from build123d import *

# Parameters (mm, degrees)
CUT_EXTRUDE1_DEPTH      = 36.362195916
CUT_EXTRUDE1_DEPTH_BACK = 36.362195916
CUT_EXTRUDE2_DEPTH      = 36.362195916
CUT_EXTRUDE2_DEPTH_BACK = 36.362195916
SKETCH4_R               = 4.245


with BuildPart() as part:
    # Sketch1 → Revolve1 (revolve)
    with BuildSketch(Plane(origin=(0, 0, 0), x_dir=(1, 0, 0), z_dir=(0, 1, 0)), mode=Mode.PRIVATE) as revolve1_sk:
        Polygon((-14, -7.07), (-14, 7.07), (-18, 7.07), (-18, 5.5), (-24.5, 5.5), (-24.5, 3.93), (-18, 3.93), (-18, 2.36), (-24.5, 2.36), (-24.5, -2.36), (-18, -2.36), (-18, -3.93), (-24.5, -3.93), (-24.5, -5.5), (-18, -5.5), (-18, -7.07), align=None)
    revolve(revolve1_sk.sketch.rotate(Axis((0, 0, 0), (0, 0, -1)), 180), axis=Axis((0, 0, 0), (0, 0, -1)))

    # Sketch3 → Cut-Extrude1 (cut, two sides: drawn at the far end of the back side and taken through both)
    with BuildSketch(Plane.XY.offset(-CUT_EXTRUDE1_DEPTH_BACK)):
        with BuildLine():
            Line((-14, 0), (-24.5, 0))
            ThreePointArc((-24.5, 0), (0, -24.5), (24.5, 0))
            Line((24.5, 0), (14, 0))
            ThreePointArc((14, 0), (0, -14), (-14, 0))
        make_face()
    extrude(amount=CUT_EXTRUDE1_DEPTH + CUT_EXTRUDE1_DEPTH_BACK, mode=Mode.SUBTRACT)

    # Sketch4 → Cut-Extrude2 (cut, two sides: drawn at the far end of the back side and taken through both)
    with BuildSketch(Plane(origin=(0, 0, 0), x_dir=(1, 0, 0), z_dir=(0, 1, 0)).offset(-CUT_EXTRUDE2_DEPTH_BACK)):
        with Locations(Location((0, 0, 0), (0, 0, 90))):
            Circle(SKETCH4_R)
    extrude(amount=CUT_EXTRUDE2_DEPTH + CUT_EXTRUDE2_DEPTH_BACK, mode=Mode.SUBTRACT)

    # Sketch6 → Tap Drill for M2x0.4 Tap1 (revolve, cut)
    with BuildSketch(Plane(origin=(-21.25, 0, 0), x_dir=(0, 0, -1), z_dir=(1, 0, 0))):
        Polygon((0, 0), (0, 7.2), (1.1, 6.564914704), (1.1, 0), align=None)
    tap_drill_for_m2x0_4_tap1 = revolve(axis=Axis((-21.25, -6.35, 0), (0, 1, 0)), mode=Mode.SUBTRACT)

    # Mirror1: Tap Drill for M2x0.4 Tap1 across plane
    add(tap_drill_for_m2x0_4_tap1.mirror(Plane(origin=(0, 0, 0), x_dir=(0, 0, 1), z_dir=(1, 0, 0))), mode=Mode.SUBTRACT)


solid = part.part
Can you work these out from the model? Positions are in its coordinate system, mm. A direction names the side the tool comes from. Coordinates: 2 decimals unless noted, no trailing zeros. Write each loop counter-clockwise with the first axis right and the second up, starting at its lowest first coordinate (ties: lowest second). Pieces come first, ordered by that corner, then holes. Notation, with made-up numbers: (76, 10.25) -> (80, 10.25) arc R28 cw to (80, 49.25) -> close; hole circle Ø9 at (-2.75, 77.5). An arc over 180 degrees is marked (long way). Write item = value, one per line.
(1) Imagine slicing it at B-B (y = 23). Please give me the cut outline in (x, z) (3 decimals), and give its area (3 significant figures).
Verdict:
outline = (-8.441, -5.5) -> (8.441, -5.5) -> (8.441, -3.93) -> (1.605, -3.93) arc R4.245 cw to (-1.605, -3.93) -> (-8.441, -3.93) -> close; (-8.441, -2.36) -> (-3.529, -2.36) arc R4.245 cw to (-3.529, 2.36) -> (-8.441, 2.36) -> close; (-8.441, 3.93) -> (-1.605, 3.93) arc R4.245 cw to (1.605, 3.93) -> (8.441, 3.93) -> (8.441, 5.5) -> (-8.441, 5.5) -> close; (3.529, -2.36) -> (8.441, -2.36) -> (8.441, 2.36) -> (3.529, 2.36) arc R4.245 cw to start
area = 93.4 mm^2
(2) Imagine slicing it at A-A (x = 0). Please give me the cut outline in (y, z) (3 decimals), and give its area (3 significant figures).
Verdict:
outline = (14, -7.07) -> (18, -7.07) -> (18, -5.5) -> (24.5, -5.5) -> (24.5, -4.245) -> (14, -4.245) -> close; (14, 4.245) -> (24.5, 4.245) -> (24.5, 5.5) -> (18, 5.5) -> (18, 7.07) -> (14, 7.07) -> close
area = 38.9 mm^2
(3) Imagine slicing it at C-C (z = 1.75). Please give me the cut outline in (x, y).
Verdict:
outline = (-24.5, 0) -> (-14, 0) arc R14 cw to (-3.87, 13.46) -> (-3.87, 24.19) arc R24.5 ccw to start; (3.87, 13.46) arc R14 cw to (14, 0) -> (24.5, 0) arc R24.5 ccw to (3.87, 24.19) -> close
(4) For pin 1 (6 mm diameter, centred on x = -9.5, z = -5.5, fed in from -Y); pin 2 (1.5 mm diameter, centred on x = -10.5, z = -3.5, fed in from -Y); pin 3 (2 mm diameter, centred on x = 21.25, z = 0, fed in from +Y); pin 4 (12 mm diameter, centred on x = 0, y = 5.5, fed in from +Z), each with a flat end and sliding along its axis, tell me the tip position at first contact or that it passes through.
Verdict:
pin_1 = 6.3
pin_2 = 8.33
pin_3 = 13.79
pin_4 = through
(5) On a 3-axis mill with a long thin cutter (end or side, diameter ignored), from which of +Z, -Z, +X, -X, +Y, -Y can I reach the whole of each face in a straight line? I mean faces 1 (the face through (20.176, 3.237, 0.238)), 2 (the face through (-16, 12, -2.36)), 3 (the face through (0, 18, -6)). Say none if no direction works.
Verdict:
face_1 = -Y
face_2 = -X, +Y
face_3 = -Z, +Y
(6) Thinking about a two-plate mould opening in X: for faces 4 (the face through (-15, 12, 3.93)), 5 (the face through (-1.275, 18.836, -4.049)), 6 (the face through (18.37, 16.21, 0.03)), which applies, +X half, -X half, draft (parallel to the pull), parting line (faces both ways), or undercut?
Verdict:
face_4 = draft
face_5 = undercut
face_6 = +X half
(7) If I drill on probe 1 along Z at (x, y) = (-17.5, 13.5); probe 2 along X at (y, z) = (3.5, 0); probe 3 along X at (y, z) = (4.5, 0), over which ranges is the centre line in solid material (lowest first)?
Verdict:
probe_1 = -5.5 to -3.93, -2.36 to 2.36, 3.93 to 5.5
probe_2 = -24.25 to -22.35, -20.15 to -13.56, 13.56 to 20.15, 22.35 to 24.25
probe_3 = -24.08 to -22.35, -20.15 to -13.26, 13.26 to 20.15, 22.35 to 24.08
(8) Imagine slicing it at D-D (x = 19). Please give me the cut outline in (y, z), and give its area (3 significant figures).
Verdict:
outline = (0, -5.5) -> (15.47, -5.5) -> (15.47, -3.93) -> (0, -3.93) -> close; (0, -2.36) -> (15.47, -2.36) -> (15.47, 2.36) -> (0, 2.36) -> close; (0, 3.93) -> (15.47, 3.93) -> (15.47, 5.5) -> (0, 5.5) -> close
area = 122 mm^2
